The listing builds one solid part. Answer for the finished solid, in the listing's coordinates (mm). Round coordinates to 2 decimals unless told otherwise and drop trailing zeros. Loops run counter-clockwise (first coordinate to the right, second up) from the corner with the lowest first, then second, coordinate; pieces in that order, holes last. Notation, with made-up numbers: (61, -12.5) -> (70, -12.5) arc R9 cw to (70, 0.5) -> close; hole circle Ø11 at (53.25, 37.5). An arc over 180 degrees is marked (long way). Write each question's results on one line, items separated by ' | '. Start each with the question number.
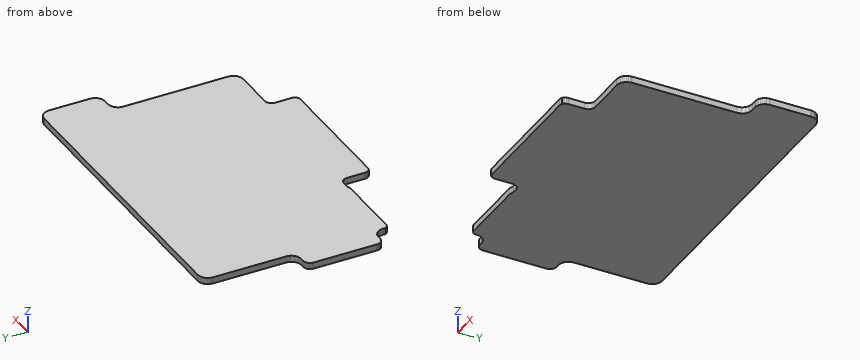
from build123d import *

# Parameters (mm, degrees)
BOSS_EXTRUDE1_DEPTH   = 0.2
BOSS_EXTRUDE1_2_DEPTH = 0.2


with BuildPart() as part:
    # Model → Boss-Extrude1 (new body)
    with BuildSketch(Plane.XY):
        Polygon((16.018, -7.896828787), (16.028, -7.902828787), (21.022, -11.541828787), (21.056, -11.580828787), (21.117, -11.686828787), (21.127, -11.709828787), (21.154, -11.790828787), (21.16, -11.845828787), (21.144, -11.968828787), (21.141, -11.986828787), (21.003, -12.477828787), (21.043, -12.827828787), (21.276, -13.254828787), (21.287, -13.282828787), (21.389, -13.673828787), (21.393, -13.702828787), (21.403, -14.128828787), (21.398, -14.165828787), (21.149, -15.015828787), (21.13, -15.055828787), (20.651, -15.696828787), (20.633, -15.716828787), (20.156, -16.126828787), (20.128, -16.144828787), (19.728, -16.335828787), (19.675, -16.347828787), (19.159, -16.347828787), (19.109, -16.337828787), (18.603, -16.117828787), (18.343, -16.037828787), (17.933, -16.107828787), (17.614, -16.474828787), (17.589, -16.496828787), (16.94, -16.929828787), (16.881, -16.950828787), (14.746, -17.127828787), (14.74, -17.127828787), (10.11, -17.127828787), (10.077, -17.122828787), (9.594, -16.986828787), (9.54, -16.954828787), (8.923, -16.337828787), (8.738, -16.337828787), (8.732, -16.335828787), (-8.046, -16.335828787), (-8.113, -16.315828787), (-8.159, -16.263828787), (-8.17, -16.211828787), (-8.17, -14.262828787), (-8.151, -14.195828787), (-8.098, -14.149828787), (-8.046, -14.138828787), (8.732, -14.138828787), (8.733, -14.137828787), (8.733, -12.396828787), (8.753, -12.329828787), (8.767, -12.311828787), (9.196, -11.856828787), (9.257, -11.821828787), (9.287, -11.817828787), (11.043, -11.817828787), (11.84, -11.212828787), (11.905, -11.187828787), (11.915, -11.187828787), (13.063, -11.187828787), (13.453, -10.907828787), (15.638, -7.967828787), (15.674, -7.934828787), (15.726, -7.903828787), (15.785, -7.886828787), (15.95, -7.879828787), align=None)
    extrude(amount=BOSS_EXTRUDE1_DEPTH)


with BuildPart() as body_2:
    # Model → Boss-Extrude1 2 (new body)
    with BuildSketch(Plane.XY):
        Polygon((4.529, 3.210171213), (4.608, 3.194171213), (4.652, 3.175171213), (4.709, 3.138171213), (4.743, 3.104171213), (4.78, 3.047171213), (4.799, 3.003171213), (4.815, 2.924171213), (4.817, 2.900171213), (4.817, 1.628171213), (4.815, 1.604171213), (4.799, 1.525171213), (4.78, 1.481171213), (4.743, 1.424171213), (4.709, 1.390171213), (4.652, 1.352171213), (4.608, 1.334171213), (4.529, 1.318171213), (4.505, 1.316171213), (4.334, 1.316171213), (4.219, 1.293171213), (4.122, 1.228171213), (4.057, 1.131171213), (4.034, 1.016171213), (4.034, -2.260828787), (4.032, -2.284828787), (4.016, -2.363828787), (3.998, -2.408828787), (3.96, -2.464828787), (3.926, -2.498828787), (3.869, -2.536828787), (3.825, -2.554828787), (3.746, -2.570828787), (3.722, -2.572828787), (2.452, -2.572828787), (2.376, -2.588828787), (2.311, -2.631828787), (2.267, -2.696828787), (2.252, -2.772828787), (2.252, -3.291828787), (2.25, -3.315828787), (2.242, -3.355828787), (2.223, -3.400828787), (2.207, -3.424828787), (2.173, -3.458828787), (2.171, -3.459828787), (2.105, -3.480828787), (2.102, -3.480828787), (-1.915, -3.477828787), (-1.983, -3.458828787), (-2.018, -3.422828787), (-2.033, -3.400828787), (-2.052, -3.355828787), (-2.06, -3.315828787), (-2.062, -3.291828787), (-2.062, -2.727828787), (-2.078, -2.650828787), (-2.121, -2.586828787), (-2.186, -2.542828787), (-2.262, -2.527828787), (-2.417, -2.527828787), (-2.493, -2.542828787), (-2.501, -2.547828787), (-2.568, -2.568828787), (-2.57, -2.568828787), (-4.693, -2.568828787), (-4.76, -2.549828787), (-4.806, -2.496828787), (-4.817, -2.444828787), (-4.817, -2.387828787), (-4.84, -2.272828787), (-4.905, -2.175828787), (-5.002, -2.110828787), (-5.117, -2.087828787), (-5.235, -2.087828787), (-5.259, -2.085828787), (-5.299, -2.076828787), (-5.344, -2.058828787), (-5.368, -2.042828787), (-5.402, -2.008828787), (-5.418, -1.984828787), (-5.437, -1.939828787), (-5.445, -1.899828787), (-5.447, -1.875828787), (-5.447, 0.100171213), (-5.445, 0.124171213), (-5.437, 0.164171213), (-5.418, 0.209171213), (-5.402, 0.233171213), (-5.368, 0.267171213), (-5.344, 0.283171213), (-5.299, 0.302171213), (-5.259, 0.310171213), (-5.235, 0.312171213), (-5.117, 0.312171213), (-5.002, 0.335171213), (-4.905, 0.400171213), (-4.84, 0.497171213), (-4.817, 0.612171213), (-4.817, 2.900171213), (-4.815, 2.924171213), (-4.799, 3.003171213), (-4.78, 3.047171213), (-4.743, 3.104171213), (-4.709, 3.138171213), (-4.652, 3.175171213), (-4.608, 3.194171213), (-4.529, 3.210171213), (-4.505, 3.212171213), (4.505, 3.212171213), align=None)
    extrude(amount=BOSS_EXTRUDE1_2_DEPTH)


solid = body_2.part
Item 1: The part is cut by section B-B, the plane y = 2. Give the vertices of the cut face in (x, z).
Item 2: The part is cut by section A-A, the plane y = -3. Give the vertices of the cut face in (x, z).
Item 3: Straight lines are drawn through the part: L1, parallel to Y at x = -1.75, z = 0.1; L2, parallel to X at y = 2.5, z = 0.15; L3, parallel to Y at x = -3, z = 0.15. For each, find the intervals that lie inside material, in ascending order. Write a range as [from, to].
Report:
1) outline: (-4.82, 0) -> (4.82, 0) -> (4.82, 0.2) -> (-4.82, 0.2) -> close
2) outline: (-2.06, 0) -> (2.25, 0) -> (2.25, 0.2) -> (-2.06, 0.2) -> close
3) L1: y = [-3.48, 3.21] | L2: x = [-4.82, 4.82] | L3: y = [-2.57, 3.21]
